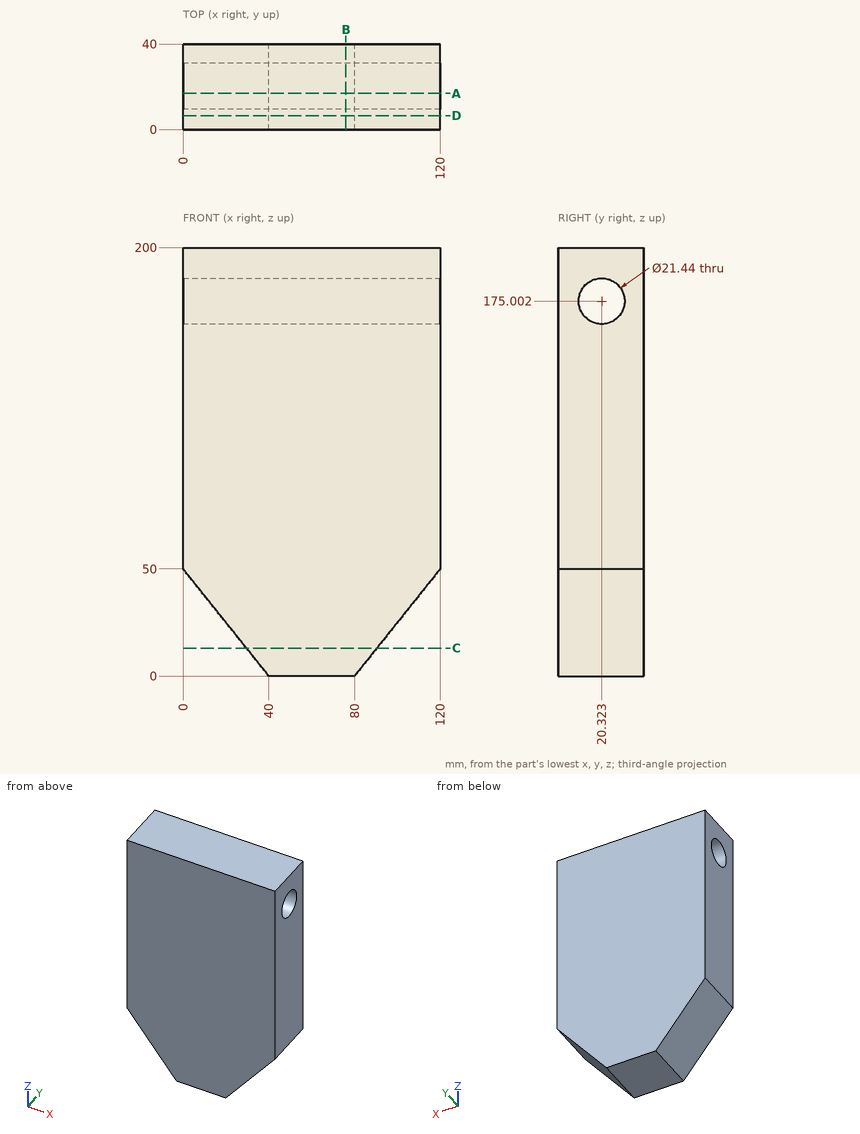
The drawing under review shows one solid part. Ordinate dimensions are in mm from its lowest x, y, z. Give positions to 0.01 mm unless a question says otherwise; leave off trailing zeros. Loops run counter-clockwise (first coordinate to the right, second up) from the corner with the lowest first, then second, coordinate; pieces in that order, holes last. Notation, with made-up numbers: M 70,40.5 L 111,40.5 A21 cw 111,57.5 Z; hole C 6.25,48 d9. An arc over 180 degrees is marked long. One line per question, with ' | ' between items. Start each with the question number.
1. Insertion check: P1, Ø8, axis at y = 27, z = 32.5, coming from the +X side; P2, Ø8, axis at x = 16.5, y = 20.5, coming from the -Z side (1 decimal); P3, Ø13, axis at y = 20.32, z = 175, coming from the -X side. Each pin has a flat end and moves straight along its axis. Give the tip position at first contact, or say it passes through.
2. Add section D-D (y = 6.5). Write out the cut boundary in (x, z).
3. Add section C-C (z = 13). Write out the cut boundary in (x, y), plus the area to 3 significant figures.
4. Add section B-B (x = 76). Write out the cut boundary in (y, z), plus the area to 3 significant figures.
5. To check wall thickness, follow L1, parallel to Z at x = 76.5, y = 17 (1 decimal); L2, parallel to Z at x = 33.5, y = 14 (1 decimal); L3, parallel to Y at x = 37, z = 180.5 (1 decimal). State the ranges of each line that lie inside material, in increasing order.
6. Add section A-A (y = 17). Write out the cut boundary in (x, z) (1 decimal), plus the area to 3 significant figures.
Worked out:
1) P1: stops at x = 109.2 | P2: stops at z = 24.4 | P3: passes through
2) outline: M 0,50 L 40,0 L 80,0 L 120,50 L 120,200 L 0,200 Z
3) outline: M 29.6,0 L 90.4,0 L 90.4,40 L 29.6,40 Z | area: 2,430 mm²
4) outline: M 0,0 L 40,0 L 40,200 L 0,200 Z; hole C 20.32,175 d21.44 | area: 7,640 mm²
5) L1: z = 0 to 164.8, 185.2 to 200 | L2: z = 8.1 to 166.3, 183.7 to 200 | L3: y = 0 to 11.1, 29.5 to 40
6) outline: M 0,50 L 40,0 L 80,0 L 120,50 L 120,164.8 L 0,164.8 Z; M 0,185.2 L 120,185.2 L 120,200 L 0,200 Z | area: 19,600 mm²
